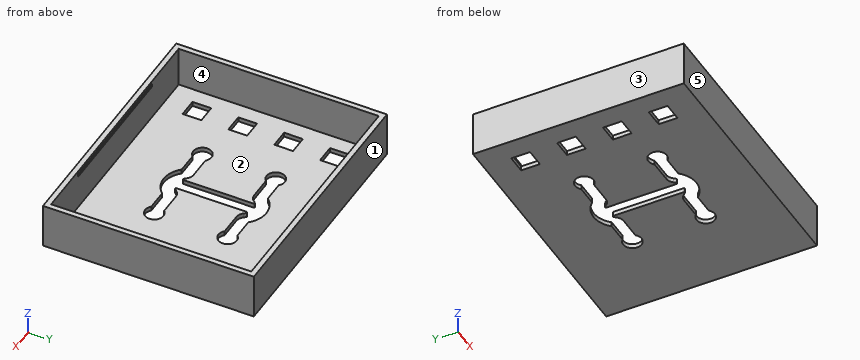
from build123d import *

# Parameters (mm, degrees)
SKETCH_1_W           = 166
SKETCH_1_H           = 138
EXTRUDE_1_DEPTH      = 3
SKETCH_2_W           = 166
SKETCH_2_H           = 138
SKETCH_2_W_2         = 159
SKETCH_2_H_2         = 131
EXTRUDE_2_DEPTH      = 27
SKETCH_3_W           = 92
SKETCH_3_H           = 2.2
CUT_EXTRUDE_1_DEPTH  = 1
SKETCH_4_W           = 92
SKETCH_4_H           = 2.2
CUT_EXTRUDE_2_DEPTH  = 1
SKETCH_11_W          = 12.3
SKETCH_11_H          = 12.3
CUT_EXTRUDE_8_DEPTH  = 10
CUT_EXTRUDE_12_DEPTH = 10
FILLET_1_R           = 6
FILLET_2_R           = 0.5


with BuildPart() as part:
    # 스케치1 → 보스-돌출1 (new body)
    with BuildSketch(Plane.XY):
        Rectangle(SKETCH_1_W, SKETCH_1_H)
    extrude(amount=EXTRUDE_1_DEPTH)

    # 스케치2 → 보스-돌출2 (add)
    with BuildSketch(Plane.XY.offset(3)):
        Rectangle(SKETCH_2_W, SKETCH_2_H)
        Rectangle(SKETCH_2_W_2, SKETCH_2_H_2, mode=Mode.SUBTRACT)
    extrude(amount=EXTRUDE_2_DEPTH)

    # 스케치3 → 컷-돌출1 (cut)
    with BuildSketch(Plane.XZ.offset(-65.5)):
        with Locations((0, 27)):
            Rectangle(SKETCH_3_W, SKETCH_3_H)
    extrude(amount=-CUT_EXTRUDE_1_DEPTH, mode=Mode.SUBTRACT)

    # 스케치4 → 컷-돌출2 (cut)
    with BuildSketch(Plane(origin=(0, -65.5, 0), x_dir=(1, 0, 0), z_dir=(0, 1, 0))):
        with Locations((0, -27)):
            Rectangle(SKETCH_4_W, SKETCH_4_H)
    extrude(amount=-CUT_EXTRUDE_2_DEPTH, mode=Mode.SUBTRACT)

    # 스케치11 → 컷-돌출8 (cut)
    with BuildSketch(Plane(origin=(0, 0, 0), x_dir=(-1, 0, 0), z_dir=(0, 0, -1))):
        with Locations((63.15, 15)):
            Rectangle(SKETCH_11_W, SKETCH_11_H)
        with Locations((63.15, 45)):
            Rectangle(SKETCH_11_W, SKETCH_11_H)
        with Locations((63.15, -15)):
            Rectangle(SKETCH_11_W, SKETCH_11_H)
        with Locations((63.15, -45)):
            Rectangle(SKETCH_11_W, SKETCH_11_H)
    extrude(amount=-CUT_EXTRUDE_8_DEPTH, mode=Mode.SUBTRACT)

    # 스케치15 → 컷-돌출12 (cut)
    with BuildSketch(Plane(origin=(0, 0, 0), x_dir=(-1, 0, 0), z_dir=(0, 0, -1))):
        with BuildLine():
            ThreePointArc((25.715142943, -28.2), (36, -24), (25.715142943, -19.8))
            Line((25.715142943, -19.8), (7.573331842, -19.8))
            ThreePointArc((7.573331842, -19.8), (6.273579039, -22.186370807), (4.25, -24))
            Line((4.25, -24), (4.25, 24))
            ThreePointArc((4.25, 24), (6.273579039, 22.186370807), (7.573331842, 19.8))
            Line((7.573331842, 19.8), (25.715142943, 19.8))
            ThreePointArc((25.715142943, 19.8), (36, 24), (25.715142943, 28.2))
            Line((25.715142943, 28.2), (12.183991333, 28.2))
            ThreePointArc((12.183991333, 28.2), (0, 33.622279144), (-12.183991333, 28.2))
            Line((-12.183991333, 28.2), (-25.715142943, 28.2))
            ThreePointArc((-25.715142943, 28.2), (-36, 24), (-25.715142943, 19.8))
            Line((-25.715142943, 19.8), (-7.573331842, 19.8))
            ThreePointArc((-7.573331842, 19.8), (-6.273579039, 22.186370807), (-4.25, 24))
            Line((-4.25, 24), (-4.25, -24))
            ThreePointArc((-4.25, -24), (-6.273579039, -22.186370807), (-7.573331842, -19.8))
            Line((-7.573331842, -19.8), (-25.715142943, -19.8))
            ThreePointArc((-25.715142943, -19.8), (-36, -24), (-25.715142943, -28.2))
            Line((-25.715142943, -28.2), (-12.183991333, -28.2))
            ThreePointArc((-12.183991333, -28.2), (0, -33.622279144), (12.183991333, -28.2))
            Line((12.183991333, -28.2), (25.715142943, -28.2))
        make_face()
    extrude(amount=-CUT_EXTRUDE_12_DEPTH, mode=Mode.SUBTRACT)

    # 필렛1
    fillet_1_edges = [part.edges().sort_by_distance(p)[0] for p in [
        (7.573331842, -19.8, 1.5),
        (-7.573331842, -19.8, 1.5),
        (7.573331842, 19.8, 1.5),
        (-7.573331842, 19.8, 1.5),
    ]]
    fillet(fillet_1_edges, radius=FILLET_1_R)

    # 필렛2
    fillet_2_edges = [part.edges().sort_by_distance(p)[0] for p in [
        (-4.25, -24, 1.5),
        (4.25, 24, 1.5),
        (4.25, -24, 1.5),
        (-4.25, 24, 1.5),
    ]]
    fillet(fillet_2_edges, radius=FILLET_2_R)


solid = part.part
Input: part model. Units: mm. Frame: model coordinates. Face numbers are marked on the shaded views. A direction names the side the tool comes from. Coordinates: 2 decimals unless noted, no trailing zeros. Loops run counter-clockwise (first coordinate to the right, second up) from the corner with the lowest first, then second, coordinate; pieces in that order, holes last.
(1) Set-up query: the marked faces 4 and 5. Return all of +Z, -Z, +X, -X, +Y, -Y with unobstructed straight access to the full face (end or side cutting, diameter ignored); none if empty.
(2) Pull-direction query (X, two-part tool) for the marked faces 1, 2 and 3; classes: released by +X, released by -X, zero draft, split by the parting line, or undercut.
(3) Section D-D on y = -54. Return the cut outline in (x, z).
(4) Section C-C on z = 22.25. Return the cut outline in (x, y), then the cut area to 3 significant figures.
(5) Material intervals for probe 1 along Y at (x, z) = (30, 1.85); probe 2 along Y at (x, z) = (-51.5, 5.5); probe 3 along X at (y, z) = (44, 2.25), sorted ascending.
(6) First-contact query: pin 1 Ø1 at (x, y) = (65.5, -45) entering from +Z. Flat tip, straight axial feed; report the tip coordinate or a pass-through.
(7) Section A-A on x = -30. Return the cut outline in (y, z), then the cut area to 3 significant figures.
(8) Section B-B on y = 16. Return the cut outline in (x, z), then the cut area to 3 significant figures.
Data:
1. face 4: +Z
1. face 5: +Z, -Z, +X, -X, -Y
2. face 1: zero draft
2. face 2: undercut
2. face 3: released by -X
3. outline: (-83, 0) - (83, 0) - (83, 30) - (79.5, 30) - (79.5, 3) - (-79.5, 3) - (-79.5, 30) - (-83, 30) - close
4. outline: (-83, -69) - (83, -69) - (83, 69) - (-83, 69) - close; hole (-79.5, -65.5) - (79.5, -65.5) - (79.5, 65.5) - (-79.5, 65.5) - close
4. area: 2,080 mm2
5. probe 1: y = -69 to -30, -18 to 18, 30 to 69
5. probe 2: y = -69 to -65.5, 65.5 to 69
5. probe 3: x = -83 to -69.3, -57 to 83
6. pin 1: stops at z = 3
7. outline: (-69, 0) - (-30, 0) - (-30, 3) - (-65.5, 3) - (-65.5, 25.9) - (-66.5, 25.9) - (-66.5, 28.1) - (-65.5, 28.1) - (-65.5, 30) - (-69, 30) - close; (-18, 0) - (18, 0) - (18, 3) - (-18, 3) - close; (30, 0) - (69, 0) - (69, 30) - (65.5, 30) - (65.5, 28.1) - (66.5, 28.1) - (66.5, 25.9) - (65.5, 25.9) - (65.5, 3) - (30, 3) - close
7. area: 527 mm2
8. outline: (-83, 0) - (-69.3, 0) - (-69.3, 3) - (-79.5, 3) - (-79.5, 30) - (-83, 30) - close; (-57, 0) - (-4.25, 0) - (-4.25, 3) - (-57, 3) - close; (4.25, 0) - (83, 0) - (83, 30) - (79.5, 30) - (79.5, 3) - (4.25, 3) - close
8. area: 625 mm2
